Answer from the drawing. Dimensions are ordinates in mm from the lowest x, y and z of the part. A direction names the side the tool comes from. Coordinates: 2 decimals unless noted, no trailing zeros. Write each loop counter-clockwise with the first axis right and the second up, starting at its lowest first coordinate (ties: lowest second). Pieces come first, ordered by that corner, then holes.
(1) The part is cut by section A-A, the plane y = 23. Determine the outline of the cut face in (x, z).
(2) Straight lines are drawn through the part: line 1 along Y through (x, z) = (27, 55); line 2 along X through (y, z) = (34, 13); line 3 along X through (y, z) = (3.5, 13). For each, find the intervals that lie inside material, in ascending order.
(3) Which of the six approach directions +Z, -Z, +X, -X, +Y, -Y give full straight-line access (tool end or side, diameter ignored) to the marked faces 4, 5 and 6?
(4) The part is cut by section B-B, the plane x = 16. Determine the outline of the cut face in (y, z).
(5) Determine the mould class of the marked faces 1, 2 and 3 for opening direction Y: pulls with the +Y half, pulls with the -Y half, needs draft (parallel to the pull), parting line crosses it, or undercut.
(6) Given pin 1 (12 mm diameter, centred on x = 86.5, y = 9.5, fed in from -Z); pin 2 (7.5 mm diameter, centred on y = 6, z = 8, fed in from +X); pin 3 (4.5 mm diameter, centred on y = 24, z = 49, fed in from -X), each flat-ended and moving along its own axis, determine where each tip first touches the part or whether it passes through.
(7) The part is cut by section D-D, the plane y = 11. Determine the outline of the cut face in (x, z), and give its area (3 significant figures).
(8) The part is cut by section C-C, the plane z = 8.5. Determine the outline of the cut face in (x, y).
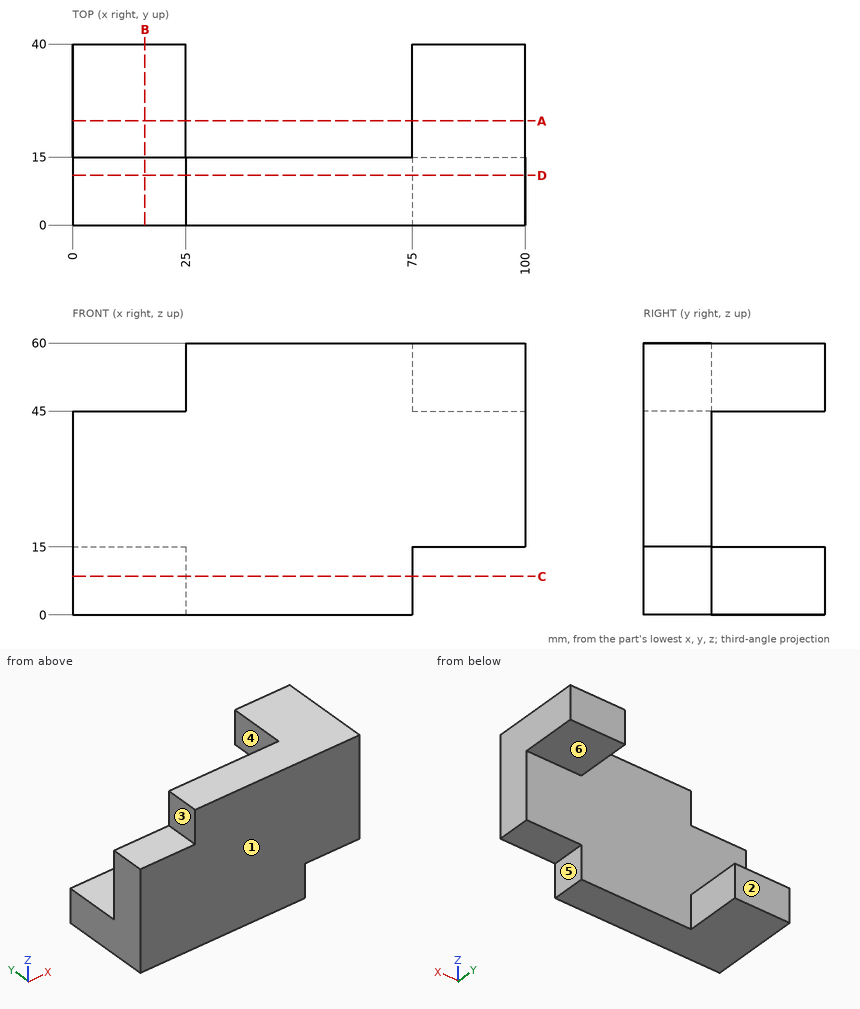
Computed:
1. outline: (0, 0) - (25, 0) - (25, 15) - (0, 15) - close; (75, 45) - (100, 45) - (100, 60) - (75, 60) - close
2. line 1: y = 0 to 15
2. line 2: x = 0 to 25
2. line 3: x = 0 to 75
3. face 4: +Z, -Z, -X, +Y
3. face 5: -Z, +X, +Y, -Y
3. face 6: -Z, +X, -X, +Y
4. outline: (0, 0) - (40, 0) - (40, 15) - (15, 15) - (15, 45) - (0, 45) - close
5. face 1: pulls with the -Y half
5. face 2: pulls with the +Y half
5. face 3: needs draft
6. pin 1: stops at z = 15
6. pin 2: stops at x = 75
6. pin 3: stops at x = 75
7. outline: (0, 0) - (75, 0) - (75, 15) - (100, 15) - (100, 60) - (25, 60) - (25, 45) - (0, 45) - close
7. area: 5,250 mm2
8. outline: (0, 0) - (75, 0) - (75, 15) - (25, 15) - (25, 40) - (0, 40) - close
